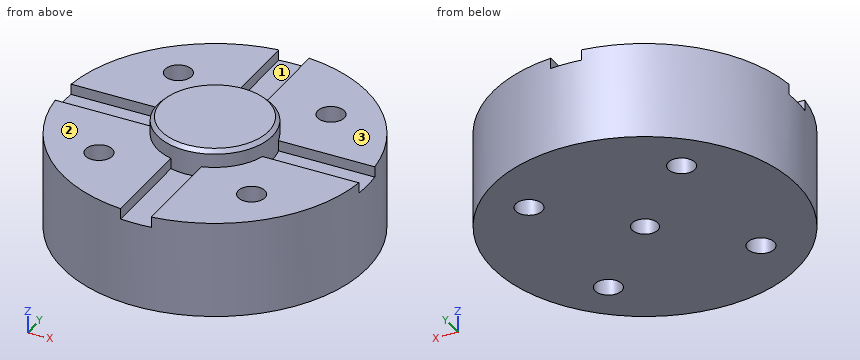
Autodesk Fusion 360 part; units mm, degrees
sketch "Skizze1" plane through (0, 0, 0) normal (0, 0, 1) x (1, 0, 0)
  circle A0 centre (0, 0) radius 20
  circle A1 centre (0, 0) radius 1.7
  line L0 (0, 23) -> (0, -24.4681) construction
  circle A2 centre (0, 0) radius 7.55
  line L1 (24, 0) -> (-23.5704, 0) construction
  line L2 (-23.8139, 10) -> (38.4686, 10) construction
  line L3 (-25.6457, -10) -> (29, -10) construction
  line L4 (-10, 25.6893) -> (-10, -22.4618) construction
  line L5 (10, 21.0661) -> (10, -25) construction
  circle A3 centre (-10, 10) radius 1.75
  circle A4 centre (10, 10) radius 1.75
  circle A5 centre (10, -10) radius 1.75
  circle A6 centre (-10, -10) radius 1.75
  line L6 (-2, 19.8997) -> (-2, -19.8997)
  line L7 (2, 19.8997) -> (2, -19.8997)
  line L8 (-19.8997, 2) -> (19.8997, 2)
  line L9 (-19.8997, -2) -> (19.8997, -2)
  point P0 (-10, 10)
  point P1 (10, 10)
  point P2 (10, -10)
  point P3 (-10, -10)
  dimension "d1" = 40
  dimension "d2" = 3.4
  dimension "d25" = 15.1
  dimension "d69" = 10
  dimension "d70" = 10
  dimension "d71" = 10
  dimension "d72" = 10
  dimension "d73" = 3.5
  dimension "d74" = 3.5
  dimension "d75" = 3.5
  dimension "d76" = 3.5
  dimension "d85" = 2
  dimension "d86" = 2
  dimension "d87" = 2
  dimension "d88" = 2
extrude "Extrusion1" add sketch "Skizze1" along normal blind 15 contours A2 L7 L8 | A2 L7 L8 L9 | A2 L7 L9 | A2 L6 L7 L8 | L6 L7 L8 L9 | A2 L6 L7 L9 | A2 L6 L8 | A2 L6 L8 L9 | A2 L6 L9 | A1
extrude "Extrusion2" cut sketch "Skizze1" along normal blind 14 contours A1
extrude "Extrusion5" add sketch "Skizze1" along normal blind 12.7 contours A0 A2 L7 L8 | A0 A2 L7 L9 | A0 A2 L6 L8 | A0 A2 L6 L9
extrude "Extrusion11" add sketch "Skizze1" along normal blind 11.3 contours A0 A2 L8 L9 | A0 A2 L6 L7 | A0 A2 L6 L7 | A0 A2 L8 L9
ref_plane "Arbeitsebene1" through (0, 0, 7.5) normal (0, 0, -1) x (-1, 0, 0)
sketch "Skizze2" plane through (0, 0, 7.5) normal (0, 0, -1) x (-1, 0, 0)
  line L0 (0, 19.4975) -> (0, -17.4097) construction
  line L1 (-20.2047, 0) -> (24.515, 0) construction
  line L2 (11, 10) -> (-11.3533, 10) construction
  line L3 (11, -10) -> (-11, -10) construction
  line L4 (10, 11.7482) -> (10, -12.1179) construction
  line L5 (-10, 11.5155) -> (-10, -12.3496) construction
  line L6 (11.6454, 7.15) -> (13.2909, 10)
  line L7 (13.2909, 10) -> (11.6454, 12.85)
  line L8 (11.6454, 12.85) -> (8.3546, 12.85)
  line L9 (8.3546, 12.85) -> (6.7091, 10)
  line L10 (6.7091, 10) -> (8.3546, 7.15)
  line L11 (8.3546, 7.15) -> (11.6454, 7.15)
  line L12 (-8.3546, 7.15) -> (-6.7091, 10)
  line L13 (-6.7091, 10) -> (-8.3546, 12.85)
  line L14 (-8.3546, 12.85) -> (-11.6454, 12.85)
  line L15 (-11.6454, 12.85) -> (-13.2909, 10)
  line L16 (-13.2909, 10) -> (-11.6454, 7.15)
  line L17 (-11.6454, 7.15) -> (-8.3546, 7.15)
  line L18 (-11.6454, -7.15) -> (-13.2909, -10)
  line L19 (-13.2909, -10) -> (-11.6454, -12.85)
  line L20 (-11.6454, -12.85) -> (-8.3546, -12.85)
  line L21 (-8.3546, -12.85) -> (-6.7091, -10)
  line L22 (-6.7091, -10) -> (-8.3546, -7.15)
  line L23 (-8.3546, -7.15) -> (-11.6454, -7.15)
  line L24 (8.3546, -7.15) -> (6.7091, -10)
  line L25 (6.7091, -10) -> (8.3546, -12.85)
  line L26 (8.3546, -12.85) -> (11.6454, -12.85)
  line L27 (11.6454, -12.85) -> (13.2909, -10)
  line L28 (13.2909, -10) -> (11.6454, -7.15)
  line L29 (11.6454, -7.15) -> (8.3546, -7.15)
  point P0 (10, 10)
  point P1 (-10, 10)
  point P2 (-10, -10)
  point P3 (10, -10)
  dimension "d77" = 10
  dimension "d78" = 10
  dimension "d79" = 10
  dimension "d80" = 10
  dimension "d81" = 5.7
  dimension "d82" = 5.7
  dimension "d83" = 5.7
  dimension "d84" = 5.7
extrude "Extrusion4" cut sketch "Skizze2" along normal blind 2.6
chamfer "Fase2" distance 0.5 angle 45 1 edges at (-7.0391, -2.7302, 15)
For this review, take the finished solid that the model builds, in its own axes (mm). Face numbers are marked on the shaded views. A direction names the side the tool comes from. Round coordinates to 2 decimals unless told otherwise and drop trailing zeros. Write each loop counter-clockwise with the first axis right and the second up, starting at its lowest first coordinate (ties: lowest second). Pieces come first, ordered by that corner, then holes. Notation, with made-up numbers: (22, 34) -> (80, 34) arc R22 cw to (80, 59) -> close; hole circle Ø9 at (67.25, -20.75). An arc over 180 degrees is marked (long way). Use one line per item in the form item = value.
Q1. To check wall thickness, follow probe 1 along Y at (x, z) = (10, 3.25); probe 2 along Y at (x, z) = (0, 7.5); probe 3 along X at (y, z) = (10, 11.4). State the ranges of each line that lie inside material, in increasing order. Write a range as from..to.
Resolved:
probe_1 = -17.32..-11.75, -8.25..8.25, 11.75..17.32
probe_2 = -20..-1.7, 1.7..20
probe_3 = -17.32..-11.75, -8.25..-2, 2..8.25, 11.75..17.32
Q2. Machinability: for the marked faces 1, 2 and 3, which of the approach directions +Z, -Z, +X, -X, +Y, -Y give a long, thin tool a straight path to every point of the face, cutting with its end or side? Answer none if there is none.
Resolved:
face_1 = +Z, +Y
face_2 = +Z, -X, -Y
face_3 = +Z, +X, +Y
Q3. Consider section B-B (x = 0). State the section outline as (y, z) points, then the cut area to 3 significant figures.
Resolved:
outline = (-20, 0) -> (-1.7, 0) -> (-1.7, 14) -> (1.7, 14) -> (1.7, 0) -> (20, 0) -> (20, 11.3) -> (7.55, 11.3) -> (7.55, 14.5) -> (7.05, 15) -> (-7.05, 15) -> (-7.55, 14.5) -> (-7.55, 11.3) -> (-20, 11.3) -> close
area = 460 mm²
Q4. Consider section C-C (z = 6.5). State the section outline as (x, y) points, then the cut area to 3 significant figures.
Resolved:
outline = circle Ø40 at (0, 0); hole (-13.29, -10) -> (-11.65, -12.85) -> (-8.35, -12.85) -> (-6.71, -10) -> (-8.35, -7.15) -> (-11.65, -7.15) -> close; hole (-13.29, 10) -> (-11.65, 7.15) -> (-8.35, 7.15) -> (-6.71, 10) -> (-8.35, 12.85) -> (-11.65, 12.85) -> close; hole circle Ø3.4 at (0, 0); hole (6.71, -10) -> (8.35, -12.85) -> (11.65, -12.85) -> (13.29, -10) -> (11.65, -7.15) -> (8.35, -7.15) -> close; hole (6.71, 10) -> (8.35, 7.15) -> (11.65, 7.15) -> (13.29, 10) -> (11.65, 12.85) -> (8.35, 12.85) -> close
area = 1,140 mm²
Q5. Clearance check with flat-ended pins moving along their axes: pin 1 Ø1.1 at (x, z) = (-14, 12) entering from -Y; pin 2 Ø6 at (x, y) = (-11, 6.5) entering from +Z; pin 3 Ø3 at (x, z) = (10, 6.5) entering from +Y. State where each tip first meets the part, or that it passes through.
Resolved:
pin_1 = -14.8
pin_2 = 12.7
pin_3 = 18.1
Q6. Consider section D-D (y = -14). State the section outline as (x, z) points, then the cut area to 3 significant figures.
Resolved:
outline = (-14.28, 0) -> (14.28, 0) -> (14.28, 12.7) -> (2, 12.7) -> (2, 11.3) -> (-2, 11.3) -> (-2, 12.7) -> (-14.28, 12.7) -> close
area = 357 mm²
Q7. Consider section A-A (x = -9.5). State how many separate pieces and enclosed holes the cut face has, then the cut area to 3 significant figures.
Resolved:
separate_pieces = 3
enclosed_holes = 0
area = 344 mm²
